from build123d import *

# Parameters (mm, degrees)
BOSS_EXTRUDE1_DEPTH   = 100
BOSS_EXTRUDE2_DEPTH   = 10
BOSS_EXTRUDE2_DRAFT   = 45
SKETCH3_R             = 34
BOSS_EXTRUDE3_DEPTH   = 10
SKETCH4_R             = 31
BOSS_EXTRUDE4_DEPTH   = 30
SKETCH5_R             = 2.5
SKETCH5_R_2           = 1.75
BOSS_EXTRUDE5_DEPTH   = 3.5
CIRPATTERN1_COUNT     = 12
BOSS_EXTRUDE6_DEPTH   = 100
SKETCH10_R            = 42.5
BOSS_EXTRUDE10_DEPTH  = 10.5
BOSS_EXTRUDE11_DEPTH  = 30
BOSS_EXTRUDE12_DEPTH  = 40
CUT_EXTRUDE1_DEPTH    = 40
SKETCH14_R            = 15
BOSS_EXTRUDE13_DEPTH  = 25
SKETCH15_R            = 15
CUT_EXTRUDE2_DEPTH    = 20
SKETCH19_R            = 15
BOSS_EXTRUDE15_DEPTH  = 5
SKETCH16_R            = 9
BOSS_EXTRUDE16_DEPTH  = 180
BODY_MOVE_COPY2_ANGLE = 180
BODY_MOVE_COPY3_ANGLE = 180


with BuildPart() as part:
    # Sketch1 → Boss-Extrude1 (new body)
    with BuildSketch(Plane(origin=(0, 0, 0), x_dir=(0, 0, -1), z_dir=(1, 0, 0))):
        with BuildLine():
            Line((-37.5, 45), (37.5, 45))
            ThreePointArc((37.5, 45), (45.880962103, 0), (37.5, -45))
            Line((37.5, -45), (-37.5, -45))
            ThreePointArc((-37.5, -45), (-45.880962103, 0), (-37.5, 45))
        make_face()
    extrude(amount=BOSS_EXTRUDE1_DEPTH)


with BuildPart() as boss_extrude2_tool:
    # Sketch2 → Boss-Extrude2 (with draft: the straight prism first)
    with BuildSketch(Plane(origin=(100, 0, 0), x_dir=(0, 0, -1), z_dir=(1, 0, 0))):
        with BuildLine():
            Line((37.5, 45), (-37.5, 45))
            ThreePointArc((-37.5, 45), (-45.880962103, 0), (-37.5, -45))
            Line((-37.5, -45), (37.5, -45))
            ThreePointArc((37.5, -45), (45.880962103, 0), (37.5, 45))
        make_face()
    extrude(amount=BOSS_EXTRUDE2_DEPTH)
    # Boss-Extrude2: the draft: its side faces are tilted about the plane it starts from
    boss_extrude2_sides = [boss_extrude2_tool.faces().sort_by_distance(p)[0] for p in [
        (105, 45, 0),
        (105, 0, 45.880962103),
        (105, -45, 0),
        (105, 0, -45.880962103),
    ]]
    draft(boss_extrude2_sides, Plane(origin=(100, 0, 0), x_dir=(0, 0, -1), z_dir=(1, 0, 0)), BOSS_EXTRUDE2_DRAFT)


with BuildPart() as part_1:
    add(part.part)

    # Boss-Extrude2: add boss_extrude2_tool
    add(boss_extrude2_tool.part)

    # Sketch3 → Boss-Extrude3 (add)
    with BuildSketch(Plane(origin=(110, 0, 0), x_dir=(0, 0, -1), z_dir=(1, 0, 0))):
        Circle(SKETCH3_R)
    extrude(amount=BOSS_EXTRUDE3_DEPTH)

    # Sketch4 → Boss-Extrude4 (add)
    with BuildSketch(Plane(origin=(120, 0, 0), x_dir=(0, 0, -1), z_dir=(1, 0, 0))):
        Circle(SKETCH4_R)
    extrude(amount=BOSS_EXTRUDE4_DEPTH)

    # Sketch5 → Boss-Extrude5 (add)
    with BuildSketch(Plane(origin=(150, 0, 0), x_dir=(0, 0, -1), z_dir=(1, 0, 0))):
        with Locations((27, 0)):
            Circle(SKETCH5_R)
        with Locations((27, 0)):
            Circle(SKETCH5_R_2, mode=Mode.SUBTRACT)
    boss_extrude5 = extrude(amount=BOSS_EXTRUDE5_DEPTH)

    # CirPattern1: Boss-Extrude5 ×12 about axis
    cirpattern1_axis = Axis((0, 0, 0.17674784), (1, 0, 0))
    for i in range(1, CIRPATTERN1_COUNT):
        add(boss_extrude5.rotate(cirpattern1_axis, i * 360 / CIRPATTERN1_COUNT))

    # Sketch6 → Boss-Extrude6 (add)
    with BuildSketch(Plane(origin=(150, 0, 0), x_dir=(0, 0, -1), z_dir=(1, 0, 0))):
        with BuildLine():
            Line((16, 0), (16, 17))
            ThreePointArc((16, 17), (0, 23.900331129), (-16, 17))
            Line((-16, 17), (-16, 0))
            Line((-16, 0), (-16, -17))
            ThreePointArc((-16, -17), (0, -23.900331129), (16, -17))
            Line((16, -17), (16, 0))
        make_face()
    extrude(amount=BOSS_EXTRUDE6_DEPTH)

    # Sketch10 → Boss-Extrude10 (add, symmetric)
    with BuildSketch(Plane.XY.offset(37.5)):
        with Locations((50, -45)):
            Circle(SKETCH10_R)
    extrude(amount=BOSS_EXTRUDE10_DEPTH, both=True)

    # Sketch11 → Boss-Extrude11 (add)
    with BuildSketch(Plane(origin=(0, 0, 27), x_dir=(-1, 0, 0), z_dir=(0, 0, -1))):
        with BuildLine():
            Line((-50, -45), (-70, -45))
            Line((-70, -45), (-70, -75))
            ThreePointArc((-70, -75), (-50, -82.639320225), (-30, -75))
            Line((-30, -75), (-30, -45))
            Line((-30, -45), (-50, -45))
        make_face()
    extrude(amount=BOSS_EXTRUDE11_DEPTH)

    # Sketch12 → Boss-Extrude12 (add)
    with BuildSketch(Plane(origin=(70, 0, 0), x_dir=(0, 0, -1), z_dir=(1, 0, 0))):
        with BuildLine():
            Line((3, -45), (3, -87))
            ThreePointArc((3, -87), (20.421855105, -68.929675658), (28, -45))
            Line((28, -45), (3, -45))
        make_face()
    extrude(amount=-BOSS_EXTRUDE12_DEPTH)

    # Sketch13 → Cut-Extrude1 (cut)
    with BuildSketch(Plane.XY.offset(-3)):
        with BuildLine():
            Line((30, -75), (30, -87))
            Line((30, -87), (70, -87))
            Line((70, -87), (70, -75))
            ThreePointArc((70, -75), (50, -82.639320225), (30, -75))
        make_face()
    extrude(amount=-CUT_EXTRUDE1_DEPTH, mode=Mode.SUBTRACT)

    # Sketch14 → Boss-Extrude13 (add)
    with BuildSketch(Plane(origin=(250, 0, 0), x_dir=(0, 0, -1), z_dir=(1, 0, 0))):
        with BuildLine():
            Line((-40, 35), (10, 35))
            ThreePointArc((10, 35), (24.142135624, 29.142135624), (30, 15))
            Line((30, 15), (30, -55))
            ThreePointArc((30, -55), (24.142135624, -69.142135624), (10, -75))
            Line((10, -75), (-40, -75))
            ThreePointArc((-40, -75), (-54.142135624, -69.142135624), (-60, -55))
            Line((-60, -55), (-60, 15))
            ThreePointArc((-60, 15), (-54.142135624, 29.142135624), (-40, 35))
        make_face()
        with Locations((-28, -45)):
            Circle(SKETCH14_R, mode=Mode.SUBTRACT)
    extrude(amount=BOSS_EXTRUDE13_DEPTH)

    # Sketch15 → Cut-Extrude2 (cut)
    with BuildSketch(Plane.XY.offset(48)):
        with Locations((50, -45)):
            Circle(SKETCH15_R)
    extrude(amount=-CUT_EXTRUDE2_DEPTH, mode=Mode.SUBTRACT)

    # Sketch19 → Boss-Extrude15 (add)
    with BuildSketch(Plane.ZY.offset(-250)):
        with Locations((28, -45)):
            Circle(SKETCH19_R)
    extrude(amount=-BOSS_EXTRUDE15_DEPTH)

    # Sketch16 → Boss-Extrude16 (add)
    with BuildSketch(Plane(origin=(70, 0, 0), x_dir=(0, 0, -1), z_dir=(1, 0, 0))):
        with Locations((-16, -59)):
            Circle(SKETCH16_R)
        with Locations((11, -59)):
            Circle(SKETCH16_R)
    extrude(amount=BOSS_EXTRUDE16_DEPTH)


with BuildPart() as part_2:
    # Body-Move/Copy1: moved
    add(part_1.part.moved(Location((-50, 45, -28))))


with BuildPart() as part_3:
    # Body-Move/Copy2: moved
    add(part_2.part.rotate(Axis((0, 0, 0), (0, 1, 0)), BODY_MOVE_COPY2_ANGLE))


with BuildPart() as part_4:
    # Body-Move/Copy3: moved
    add(part_3.part.rotate(Axis((0, 0, 0), (0, 0, 1)), BODY_MOVE_COPY3_ANGLE))


solid = part_4.part
Read the model definition and answer for the solid it produces. Units are mm, in the model's axes. A direction names the side the tool comes from. Round coordinates to 2 decimals unless told otherwise and drop trailing zeros. Write each loop counter-clockwise with the first axis right and the second up, starting at its lowest first coordinate (ties: lowest second). Pieces come first, ordered by that corner, then holes.
Q1. Straight lines are drawn through the part: line 1 (Z direction, x = 102, y = -45); line 2 (X direction, y = -22, z = 19); line 3 (Y direction, x = 48.5, z = 0.5). For each, find the intervals that lie inside material, in ascending order.
Values:
line 1: z = -1.85 to -1.1, 2.4 to 3.15, 12 to 44, 52.5 to 53.25, 56.75 to 57.5
line 2: x = -50 to 100, 200 to 225
line 3: y = -90 to 0
Q2. Flat-ended cylindrical pins translate along their axes: P1, Ø1, axis at x = 80.5, y = 6.5, coming from the +Z side; P2, Ø2, axis at x = 19.5, y = -59, coming from the -Z side; P3, Ø3, axis at x = 165, y = -28, coming from the -Z side. Find the tip coordinate at first contact, or state that the pin passes through.
Values:
P1: stops at z = 44.66
P2: stops at z = -17.2
P3: stops at z = 12
Q3. A tool of negligible diameter and unlimited length cuts with its end or side. For faces 4 (the face through (101.73, -60.43, 53.05)), 5 (the face through (212, -80, 13)), 6 (the face through (-9.21, 41.49, -11.98)), 7 (the face through (103.5, -70, 40)), from which of +Z, -Z, +X, -X, +Y, -Y can it reach the whole face along a straight path? Write none if from no direction.
Values:
face 4: none
face 5: +Z, -Z, +X, -Y
face 6: -Z
face 7: +Z, -Y
Q4. Find section A-A on x = 148. Determine the outline of the cut face in (y, z), and give its area (3 significant figures).
Values:
outline: (-62, 12) - (-28, 12) arc R22 ccw to (-28, 44) - (-62, 44) arc R22 ccw to start; circle Ø18 at (14, 12); circle Ø18 at (14, 39)
area: 1,900 mm2
Q5. The mould has two halves that part along Z. Classify faces 1 (the face through (103.5, -23, 16)), 2 (the face through (56.04, -45.61, -11.84)), 3 (the face through (101.726, -33.796, 3.537)): released by +Z, released by -Z, zero draft, split by the parting line, or undercut.
Values:
face 1: zero draft
face 2: released by -Z
face 3: undercut
